The listing builds one solid part. Answer for the finished solid, in the listing's coordinates (mm). Give positions to 0.01 mm unless a question says otherwise; leave off trailing zeros. Order: outer loops, then holes, each group sorted by start corner. A loop starts at its lowest first (then second) coordinate and runs counter-clockwise, first axis right, second up.
```python
from build123d import *

# Parameters (mm, degrees)
SKETCH1_R           = 15
BOSS_EXTRUDE1_DEPTH = 0.24


with BuildPart() as part:
    # Sketch1 → Boss-Extrude1 (new body)
    with BuildSketch(Plane(origin=(0, 0, 0), x_dir=(1, 0, 0), z_dir=(0, 1, 0))):
        Polygon((0, 0), (11, 0), (14.168906797, 1.312604173), (21.94708139, 9.090778766), (23.259685563, 12.259685563), (23.259685563, 23.259685563), (21.94708139, 26.428592359), (14.168906797, 34.206766952), (11, 35.519371125), (0, 35.519371125), (-3.168906797, 34.206766952), (-10.94708139, 26.428592359), (-12.259685563, 23.259685563), (-12.259685563, 12.259685563), (-10.94708139, 9.090778766), (-3.168906797, 1.312604173), align=None)
        with Locations(Location((5.5, 17.759685563, 0), (0, 0, 270))):
            Circle(SKETCH1_R, mode=Mode.SUBTRACT)
    extrude(amount=BOSS_EXTRUDE1_DEPTH)


solid = part.part
```
1) Given P1, Ø1, axis at x = 13, z = -7, coming from the +Y side, flat-ended and moving along its own axis, determine where the tip first touches the part or whether it passes through.
Geometry says:
P1: passes through
2) Find section A-A (x = 5.5). Write down the section's boundary in (y, z).
Geometry says:
outline: (0, -35.52) - (0.24, -35.52) - (0.24, -32.76) - (0, -32.76) - close; (0, -2.76) - (0.24, -2.76) - (0.24, 0) - (0, 0) - close
3) Straight lines are drawn through the part: probe 1 along X at (y, z) = (0.1, -16.5); probe 2 along X at (y, z) = (0.2, -24.5); probe 3 along Z at (x, y) = (2.5, 0.1). For each, find the intervals that lie inside material, in ascending order.
Geometry says:
probe 1: x = -12.26 to -9.45, 20.45 to 23.26
probe 2: x = -11.75 to -7.9, 18.9 to 22.75
probe 3: z = -35.52 to -32.46, -3.06 to 0
4) Find section B-B (z = -16.5). Write down the section's boundary in (x, y).
Geometry says:
outline: (-12.26, 0) - (-9.45, 0) - (-9.45, 0.24) - (-12.26, 0.24) - close; (20.45, 0) - (23.26, 0) - (23.26, 0.24) - (20.45, 0.24) - close
5) Find section C-C (y = 0.15). Write down the section's boundary in (x, z).
Geometry says:
outline: (-12.26, -23.26) - (-10.95, -26.43) - (-3.17, -34.21) - (0, -35.52) - (11, -35.52) - (14.17, -34.21) - (21.95, -26.43) - (23.26, -23.26) - (23.26, -12.26) - (21.95, -9.09) - (14.17, -1.31) - (11, 0) - (0, 0) - (-3.17, -1.31) - (-10.95, -9.09) - (-12.26, -12.26) - close; hole circle Ø30 at (5.5, -17.76)
